from build123d import *

# Parameters (mm, degrees)
F0_R     = 9.525
F1_DEPTH = 25.4
F3_DEPTH = 25.401
F4_R     = 9.525
F5_DEPTH = 25.4
F6_W     = 9.9143758416
F6_H     = 9.589554742
F7_DEPTH = 50.801


with BuildPart() as f1:
    # F0 (on Front) → F1 (new body)
    with BuildSketch(Plane.XZ):
        Circle(F0_R)
    extrude(amount=F1_DEPTH)

    # F2 (on Front) → F3 (cut, through all)
    with BuildSketch(Plane.XZ):
        with BuildLine():
            ThreePointArc((-4.7625, 0), (-3.3675960454, -3.3675960454), (0, -4.7625))
            ThreePointArc((0, -4.7625), (3.3675960454, -3.3675960454), (4.7625, 0))
            ThreePointArc((4.7625, 0), (3.3675960454, 3.3675960454), (0, 4.7625))
            ThreePointArc((0, 4.7625), (-3.3675960454, 3.3675960454), (-4.7625, 0))
        make_face()
    extrude(amount=F3_DEPTH, mode=Mode.SUBTRACT)

    # F4 (on face) → F5 (join)
    with BuildSketch(Plane(origin=(0, 0, 0), x_dir=(-1, 0, 0), z_dir=(0, 1, 0))):
        Circle(F4_R)
        Polygon((-5.9788160654, 3.6644153505), (0.1840687509, 7.0100142725), (6.1628848163, 3.3455989219), (5.9788160654, -3.6644153505), (-0.1840687509, -7.0100142725), (-6.1628848163, -3.3455989219), align=None, mode=Mode.SUBTRACT)
    extrude(amount=F5_DEPTH)

    # F6 (on face) → F7 (cut, through all)
    with BuildSketch(Plane.XZ.offset(25.4)):
        Rectangle(F6_W, F6_H)
    extrude(amount=-F7_DEPTH, mode=Mode.SUBTRACT)


solid = f1.part
Model file for the job. Use its own axes, mm. A direction names the side the tool comes from. Give positions to 0.01 mm unless a question says otherwise; leave off trailing zeros. Loops run counter-clockwise (first coordinate to the right, second up) from the corner with the lowest first, then second, coordinate; pieces in that order, holes last.
Item 1: Mould opens along X. For faces 1 (the face through (5.55, 12.52, -3.72)), 2 (the face through (-2, 25.4, -6)), 3 (the face through (1.966, 12.522, -5.918)) say: +X half, -X half, draft (parallel to the pull), parting line (faces both ways), or undercut.
Check values:
face 1: undercut
face 2: draft
face 3: undercut
Item 2: Drill centre lines: line 1 along X through (y, z) = (-11.5, 0) (3 decimals); line 2 along Z through (x, y) = (3.5, 20.5); line 3 along Z through (x, y) = (4.75, 15). Where is each one in solid material? Low to high.
Check values:
line 1: x = -9.525 to -4.957, 4.957 to 9.525
line 2: z = -8.86 to -4.98, 5.01 to 8.86
line 3: z = -8.26 to -4.79, 4.79 to 8.26
Item 3: Slice it at A-A (y = -11). Write the cut outline in (x, z) (3 decimals).
Check values:
outline: circle Ø19.05 at (0, 0); hole (-4.957, -4.795) - (4.957, -4.795) - (4.957, 4.795) - (-4.957, 4.795) - close
Item 4: Drop flat-ended pins along their axis: P1, Ø0.7, axis at x = 0.5, z = -6, coming from the +Y side; P2, Ø2, axis at x = -6, y = -10, coming from the +Z side; P3, Ø3, axis at x = -6, y = 18, coming from the +Z side (3 decimals). Give the stop position or say it passes through.
Check values:
P1: stops at y = 0
P2: stops at z = 8.11
P3: stops at z = 8.395
Item 5: Slice it at B-B (x = 2.5). Write the cut outline in (y, z).
Check values:
outline: (-25.4, -9.19) - (25.4, -9.19) - (25.4, -5.59) - (0, -5.59) - (0, -4.79) - (-25.4, -4.79) - close; (-25.4, 4.79) - (0, 4.79) - (0, 5.55) - (25.4, 5.55) - (25.4, 9.19) - (-25.4, 9.19) - close
Item 6: Slice it at D-D (y = 9). Write the cut outline in (x, z) (3 decimals), plus the area to 3 significant figures.
Check values:
outline: circle Ø19.05 at (0, 0); hole (-6.163, 3.346) - (-5.979, -3.664) - (-4.957, -4.219) - (-4.957, -4.795) - (-3.897, -4.795) - (0.184, -7.01) - (3.798, -4.795) - (4.957, -4.795) - (4.957, -4.085) - (6.163, -3.346) - (5.979, 3.664) - (4.957, 4.219) - (4.957, 4.795) - (3.897, 4.795) - (-0.184, 7.01) - (-3.798, 4.795) - (-4.957, 4.795) - (-4.957, 4.085) - close
area: 156 mm2
Item 7: Slice it at C-C (z = 2.5). Write the cut outline in (x, y).
Check values:
outline: (-9.19, -25.4) - (-4.96, -25.4) - (-4.96, 0) - (-6.14, 0) - (-6.14, 25.4) - (-9.19, 25.4) - close; (4.96, -25.4) - (9.19, -25.4) - (9.19, 25.4) - (6.01, 25.4) - (6.01, 0) - (4.96, 0) - close
Item 8: Which spindle directions (+Z, -Z, +X, -X, +Y, -Y) get a long thin tool onto all of the face, cutting with end or side? Do faces 4 (the face through (-5.55, 12.52, 3.72)), 5 (the face through (0, -6, -4.795)), 6 (the face through (0, -25.4, -6)). Say none if no direction does.
Check values:
face 4: +Y
face 5: +Y, -Y
face 6: +Z, -Z, +X, -X, -Y
